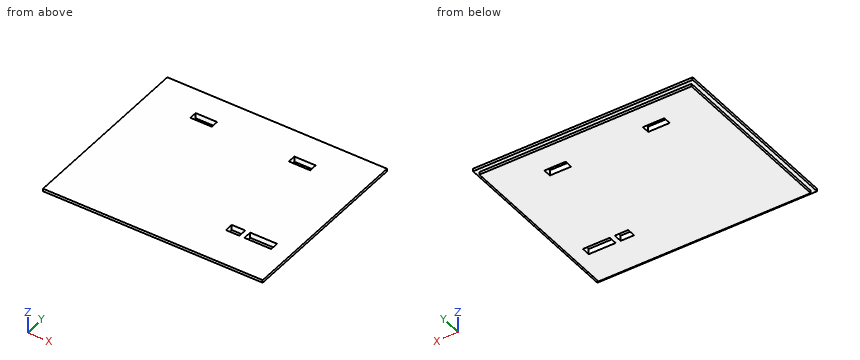
from build123d import *

# Parameters (mm, degrees)
SKETCH1_W           = 122
SKETCH1_H           = 101.3
BOSS_EXTRUDE1_DEPTH = 3
SKETCH2_W           = 1.5
SKETCH2_H           = 2.1
CUT_EXTRUDE2_DEPTH  = 130
SKETCH3_W           = 1.5
SKETCH3_H           = 2.1
CUT_EXTRUDE3_DEPTH  = 123
SKETCH4_W           = 2.1
SKETCH4_H           = 1.5
CUT_EXTRUDE4_DEPTH  = 123
SKETCH5_W           = 2.1
SKETCH5_H           = 1.5
CUT_EXTRUDE5_DEPTH  = 123
SKETCH7_W           = 7.497772187
SKETCH7_H           = 4.759480864
CUT_EXTRUDE6_DEPTH  = 5
SKETCH8_W           = 11.848959364
SKETCH8_H           = 4.476273538
CUT_EXTRUDE7_DEPTH  = 5
SKETCH9_W           = 11.911321609
SKETCH9_H           = 4.308108171
CUT_EXTRUDE8_DEPTH  = 5
SKETCH6_W           = 14.939397766
SKETCH6_H           = 4.753444744
CUT_EXTRUDE9_DEPTH  = 5


with BuildPart() as part:
    # Sketch1 → Boss-Extrude1 (new body)
    with BuildSketch(Plane.XY):
        with Locations((129.5, -82.15)):
            Rectangle(SKETCH1_W, SKETCH1_H)
    extrude(amount=BOSS_EXTRUDE1_DEPTH)

    # Sketch2 → Cut-Extrude2 (cut)
    with BuildSketch(Plane(origin=(190.5, 0, 0), x_dir=(0, 0, -1), z_dir=(1, 0, 0))):
        with Locations((-0.75, -131.75)):
            Rectangle(SKETCH2_W, SKETCH2_H)
    extrude(amount=-CUT_EXTRUDE2_DEPTH, mode=Mode.SUBTRACT)

    # Sketch3 → Cut-Extrude3 (cut)
    with BuildSketch(Plane(origin=(190.5, 0, 0), x_dir=(0, 0, -1), z_dir=(1, 0, 0))):
        with Locations((-0.75, -32.55)):
            Rectangle(SKETCH3_W, SKETCH3_H)
    extrude(amount=-CUT_EXTRUDE3_DEPTH, mode=Mode.SUBTRACT)

    # Sketch4 → Cut-Extrude4 (cut)
    with BuildSketch(Plane(origin=(0, -31.5, 0), x_dir=(1, 0, 0), z_dir=(0, 1, 0))):
        with Locations((69.55, -0.75)):
            Rectangle(SKETCH4_W, SKETCH4_H)
    extrude(amount=-CUT_EXTRUDE4_DEPTH, mode=Mode.SUBTRACT)

    # Sketch5 → Cut-Extrude5 (cut)
    with BuildSketch(Plane(origin=(0, -31.5, 0), x_dir=(1, 0, 0), z_dir=(0, 1, 0))):
        with Locations((189.45, -0.75)):
            Rectangle(SKETCH5_W, SKETCH5_H)
    extrude(amount=-CUT_EXTRUDE5_DEPTH, mode=Mode.SUBTRACT)

    # Sketch7 → Cut-Extrude6 (cut)
    with BuildSketch(Plane.XY.offset(3)):
        with Locations((159.126113906, -108.853990326)):
            Rectangle(SKETCH7_W, SKETCH7_H)
    extrude(amount=-CUT_EXTRUDE6_DEPTH, mode=Mode.SUBTRACT)

    # Sketch8 → Cut-Extrude7 (cut)
    with BuildSketch(Plane.XY.offset(3)):
        with Locations((156.118860553, -50.111595953)):
            Rectangle(SKETCH8_W, SKETCH8_H)
    extrude(amount=-CUT_EXTRUDE7_DEPTH, mode=Mode.SUBTRACT)

    # Sketch9 → Cut-Extrude8 (cut)
    with BuildSketch(Plane.XY.offset(3)):
        with Locations((100.333019396, -48.546030804)):
            Rectangle(SKETCH9_W, SKETCH9_H)
    extrude(amount=-CUT_EXTRUDE8_DEPTH, mode=Mode.SUBTRACT)

    # Sketch6 → Cut-Extrude9 (cut)
    with BuildSketch(Plane.XY.offset(3)):
        with Locations((173.124127973, -108.889085644)):
            Rectangle(SKETCH6_W, SKETCH6_H)
    extrude(amount=-CUT_EXTRUDE9_DEPTH, mode=Mode.SUBTRACT)


solid = part.part
Verification items for the finished model (mm, model axes). Give positions to 0.01 mm unless a question says otherwise; leave off trailing zeros. Order: outer loops, then holes, each group sorted by start corner. A loop starts at its lowest first (then second) coordinate and runs counter-clockwise, first axis right, second up. Notation, with made-up numbers: M 67.25,50 L 89.25,50 A29 cw 89.25,70 Z; hole C -11.75,47.5 d10. An arc over 180 degrees is marked long. Use one line per item in the form item = value. Start each with the question number.
Q1. Scan lines: line 1 along X through (y, z) = (-110, 2.5) (3 decimals); line 2 along Y through (x, z) = (94.5, 1.7); line 3 along Y through (x, z) = (155, 1.35). Record each from-to range of solid material in increasing order. Write a range as [from, to].
Q2. Section check D-D (x = 78.5). Enter the section's corners in (y, z).
Q3. Section check B-B (z = 0.65). Enter the section's corners in (x, y) (3 decimals).
Q4. Go/stop test with a flat-tipped pin: pin 1 Ø0.9 at (y, z) = (-108.5, 1) entering from -X. Record where the tip stops, or that it passes through.
Q5. Section check A-A (x = 168.5). Enter the section's corners in (y, z), then the cut area to 3 significant figures.
Q6. Section check C-C (y = -40.5). Enter the section's corners in (x, z).
Evaluation:
q1.line_1 = [68.5, 155.377], [162.875, 165.654], [180.594, 190.5]
q1.line_2 = [-132.8, -50.7], [-46.39, -31.5]
q1.line_3 = [-130.7, -52.35], [-47.87, -33.6]
q2.outline = M -132.8,1.5 L -130.7,1.5 L -130.7,0 L -33.6,0 L -33.6,1.5 L -31.5,1.5 L -31.5,3 L -132.8,3 Z
q3.outline = M 70.6,-130.7 L 188.4,-130.7 L 188.4,-33.6 L 70.6,-33.6 Z; hole M 94.377,-50.7 L 106.289,-50.7 L 106.289,-46.392 L 94.377,-46.392 Z; hole M 150.194,-52.35 L 162.043,-52.35 L 162.043,-47.873 L 150.194,-47.873 Z; hole M 155.377,-111.234 L 162.875,-111.234 L 162.875,-106.474 L 155.377,-106.474 Z; hole M 165.654,-111.266 L 180.594,-111.266 L 180.594,-106.512 L 165.654,-106.512 Z
q4.pin_1 = 70.6
q5.outline = M -132.8,1.5 L -130.7,1.5 L -130.7,0 L -111.27,0 L -111.27,3 L -132.8,3 Z; M -106.51,0 L -33.6,0 L -33.6,1.5 L -31.5,1.5 L -31.5,3 L -106.51,3 Z
q5.area = 283 mm2
q6.outline = M 68.5,1.5 L 70.6,1.5 L 70.6,0 L 188.4,0 L 188.4,1.5 L 190.5,1.5 L 190.5,3 L 68.5,3 Z
